```python
from build123d import *

# Parameters (mm, degrees)
F0_W     = 64.6
F0_H     = 136.3
F0_W_2   = 49.6
F0_H_2   = 48.8
F1_DEPTH = 13
F3_DEPTH = 57.25
F4_DEPTH = 64.6
F5_SIZE  = 2
F6_R     = 2
F7_DEPTH = 8
F6_R_2   = 4
F8_DEPTH = 5.5


with BuildPart() as f1:
    # F0 (on Top) → F1 (new body)
    with BuildSketch(Plane.XY):
        with Locations((-32.3, 15.001252)):
            Rectangle(F0_W, F0_H)
        with Locations((-30.3, -18.748748)):
            Rectangle(F0_W_2, F0_H_2, mode=Mode.SUBTRACT)
    extrude(amount=-F1_DEPTH)

    # F2 (on face) → F3 (cut)
    with BuildSketch(Plane.YZ):
        Polygon((-45.148748, -2.5), (-45.148748, -1), (-49.148748, -5), (83.151252, -5), (83.151252, -2), align=None)
    extrude(amount=-F3_DEPTH, mode=Mode.SUBTRACT)

    # F2 (on face) → F4 (cut, through all)
    with BuildSketch(Plane.YZ):
        Polygon((83.151252, 0), (-45.148748, 0), (-45.148748, -1), (-45.148748, -2.5), (83.151252, -2), align=None)
    extrude(amount=-F4_DEPTH, mode=Mode.SUBTRACT)

    # F5
    f5_edges = [f1.edges().sort_by_distance(p)[0] for p in [
        (-57.25, 19.001252, -2.25),
        (-30.3, -43.148748, -5),
        (-55.1, -18.748748, -5),
        (-30.3, 5.651252, -5),
        (-5.5, -18.748748, -5),
        (-30.3, 5.651252, -13),
        (-55.1, -18.748748, -13),
        (-30.3, -43.148748, -13),
        (-5.5, -18.748748, -13),
    ]]
    chamfer(f5_edges, length=F5_SIZE)

    # F6 (on face) → F7 (cut, through all)
    with BuildSketch(Plane.XY.offset(-5)):
        with Locations((-6, 57.651252)):
            Circle(F6_R)
        with Locations((-6, 37.651252)):
            Circle(F6_R)
        with Locations((-27, 37.651252)):
            Circle(F6_R)
        with Locations((-39, 37.651252)):
            Circle(F6_R)
        with Locations((-39, 17.651252)):
            Circle(F6_R)
        with Locations((-27, 17.651252)):
            Circle(F6_R)
    extrude(amount=-F7_DEPTH, mode=Mode.SUBTRACT)

    # F6 (on face) → F8 (cut)
    with BuildSketch(Plane.XY.offset(-5)):
        with Locations((-6, 57.651252)):
            Circle(F6_R_2)
        with Locations((-6, 57.651252)):
            Circle(F6_R, mode=Mode.SUBTRACT)
        with Locations((-6, 37.651252)):
            Circle(F6_R_2)
        with Locations((-6, 37.651252)):
            Circle(F6_R, mode=Mode.SUBTRACT)
        with Locations((-27, 37.651252)):
            Circle(F6_R_2)
        with Locations((-27, 37.651252)):
            Circle(F6_R, mode=Mode.SUBTRACT)
        with Locations((-39, 37.651252)):
            Circle(F6_R_2)
        with Locations((-39, 37.651252)):
            Circle(F6_R, mode=Mode.SUBTRACT)
        with Locations((-39, 17.651252)):
            Circle(F6_R_2)
        with Locations((-39, 17.651252)):
            Circle(F6_R, mode=Mode.SUBTRACT)
        with Locations((-27, 17.651252)):
            Circle(F6_R_2)
        with Locations((-27, 17.651252)):
            Circle(F6_R, mode=Mode.SUBTRACT)
    extrude(amount=-F8_DEPTH, mode=Mode.SUBTRACT)

    # F9: F1 across face


with BuildPart() as f1_1:
    add(f1.part)
    add(f1.part.mirror(Plane(origin=(0, 13.153307, -8.806367), x_dir=(0, 1, 0), z_dir=(1, 0, 0))))


solid = f1_1.part
```
Read the model definition and answer for the solid it produces. Units are mm, in the model's axes. A direction names the side the tool comes from. Round coordinates to 2 decimals unless told otherwise and drop trailing zeros. Write each loop counter-clockwise with the first axis right and the second up, starting at its lowest first coordinate (ties: lowest second). Pieces come first, ordered by that corner, then holes. Notation, with made-up numbers: (-11, 79) - (5, 79) arc R30 cw to (5, 108) - close; hole circle Ø1 at (-11, 65). An arc over 180 degrees is marked (long way). One line per item, written item: value.
Q1. Which of the six approach directions +Z, -Z, +X, -X, +Y, -Y give full straight-line access (tool end or side, diameter ignored) to faces 1 (the cylindrical face through (-29.95, 40.35, -7.71)), 2 (the flat face through (-31, 5.651, -9)), 3 (the flat face through (1, -53.149, -6))?
The answers:
face 1: +Z
face 2: +Z, -Z
face 3: +Z, -Z, +X, -X, -Y
Q2. Find section A-A (x = -27). Count the separate pieces of the cut face and the enclosed holes in it, and give its area (3 significant figures).
The answers:
separate pieces: 4
enclosed holes: 0
area: 616 mm2
Q3. Find section B-B (x = 50.5). Determine the outline of the cut face in (y, z).
The answers:
outline: (-53.15, -13) - (-45.15, -13) - (-43.15, -11) - (-43.15, -7) - (-45.15, -5) - (-49.15, -5) - (-45.15, -1) - (-45.15, 0) - (-53.15, 0) - close; (5.65, -11) - (7.65, -13) - (83.15, -13) - (83.15, -5) - (7.65, -5) - (5.65, -7) - close
Q4. Find section C-C (y = 44). Determine the outline of the cut face in (x, z).
The answers:
outline: (-64.6, -13) - (64.6, -13) - (64.6, -2.15) - (59.25, -2.15) - (57.25, -4.15) - (57.25, -5) - (-57.25, -5) - (-57.25, -4.15) - (-59.25, -2.15) - (-64.6, -2.15) - close
Q5. For a pull along Z with two mould halves and no side action, classify faces 4 (the flat face through (-0.8, -47.12, -2.97)), 5 (the cylindrical face through (6.521, 41.617, -7.712)), 6 (the flat face through (41, 19, -10.5)) as pulls with the +Z half, pulls with the -Z half, needs draft (parallel to the pull), parting line crosses it, or undercut.
The answers:
face 4: undercut
face 5: needs draft
face 6: pulls with the +Z half
Q6. Straight lines are drawn through the part: line 1 (Y direction, x = 6, z = -9.2); line 2 (X direction, y = -38, z = -10.25); line 3 (Y direction, x = -44, z = -8.5). For each, find the intervals that lie inside material, in ascending order. Write a range as from..to.
The answers:
line 1: y = -53.15..-43.15, 5.65..33.65, 41.65..53.65, 61.65..83.15
line 2: x = -64.6..-55.1, -5.5..5.5, 55.1..64.6
line 3: y = -53.15..-43.15, 5.65..83.15
Q7. Each of these flat-tipped pins is pushed along its axis until it touches: P1, Ø4.5, axis at x = 39, y = 17.65, coming from the +Z side; P2, Ø9, axis at x = 25, y = 18.5, coming from the +Z side; P3, Ø3, axis at x = -6, y = 57.65, coming from the -Z side. Where does it stop, or does it pass through?
The answers:
P1: stops at z = -10.5
P2: stops at z = -5
P3: passes through
